from build123d import *

# Parameters (mm, degrees)
F1_DEPTH = 10
F3_D     = 3.4
F4_R     = 3


with BuildPart() as f1:
    # F0 (on Top) → F1 (new body, symmetric)
    with BuildSketch(Plane.XY):
        with BuildLine():
            ThreePointArc((-2, -12.338963), (0, 12.5), (2, -12.338963))
            Line((2, -12.338963), (2, -25))
            Line((2, -25), (30, -25))
            Line((30, -25), (30, -15))
            Line((30, -15), (17.5, -15))
            Line((17.5, -15), (17.5, 0))
            ThreePointArc((17.5, 0), (0, 17.5), (-17.5, 0))
            Line((-17.5, 0), (-17.5, -15))
            Line((-17.5, -15), (-30, -15))
            Line((-30, -15), (-30, -25))
            Line((-30, -25), (-2, -25))
            Line((-2, -25), (-2, -12.338963))
        make_face()
    extrude(amount=F1_DEPTH, both=True)

    # F3 (through all)
    with Locations(Plane(origin=(0, -15, 0), x_dir=(-1, 0, 0), z_dir=(0, 1, 0))):
        with Locations((24, 0), (-24, 0)):
            Hole(F3_D / 2)

    # F4
    f4_edges = [f1.edges().sort_by_distance(p)[0] for p in [
        (17.5, -15, 0),
        (-17.5, -15, 0),
        (-30, -20, 10),
        (-30, -20, -10),
        (30, -20, 10),
        (30, -20, -10),
    ]]
    fillet(f4_edges, radius=F4_R)


solid = f1.part
Design review of the part built by this model. Coordinates are the model's own, in mm. A direction names the side the tool comes from. Give positions to 0.01 mm unless a question says otherwise; leave off trailing zeros. Loops run counter-clockwise (first coordinate to the right, second up) from the corner with the lowest first, then second, coordinate; pieces in that order, holes last. Notation, with made-up numbers: M 40.25,68 L 83.25,68 A27 cw 83.25,100 Z; hole C 33.5,18.25 d8. An arc over 180 degrees is marked long. One line per question, with ' | ' between items. Start each with the question number.
1. The part is to be moulded in two halves that separate along X. For faces 1 (the face through (-0.52, 12.49, 0.14)), 2 (the face through (29.1, -19.93, 9.14)), 3 (the face through (-29.1, -20.07, -9.14)), say which applies: released by +X, released by -X, zero draft, split by the parting line, or undercut.
2. To check wall thickness, follow L1, parallel to Z at x = 24, y = -16.5; L2, parallel to X at y = -15.5, z = 5.75; L3, parallel to X at y = -7.5, z = -0.25. State the ranges of each line that lie inside material, in increasing order.
3. Add section B-B (x = 24). Write out the cut boundary in (y, z), plus the area to 3 significant figures.
4. Insertion check: P1, Ø5, axis at x = -23, z = -2.5, coming from the +Y side; P2, Ø12, axis at y = -13, z = -3, coming from the -X side; P3, Ø7.5, axis at x = 23, z = -0.5, coming from the +Y side; P4, Ø4, axis at y = -2.5, z = -3, coming from the +X side. Each pin has a flat end and moves straight along its axis. Give the tip position at first contact, or say it passes through.
5. For faces 4 (the face through (2, -19, 0)), 5 (the face through (-17.5, -6, 0)), 6 (the face through (25.57, -20.07, -0.65)), 7 (the face through (17.5, -6, 0)), list the 3-axis set-ups (+Z, -Z, +X, -X, +Y, -Y) from which the entire face can be reached by the end or side of a thin tool; tool diameter is ignored.
6. Add section A-A (y = -19). Write out the cut boundary in (x, z), plus the area to 3 significant figures.
7. Add section C-C (z = 0). Write out the cut boundary in (x, y).
8. Add section D-D (z = 5.25). Write out the cut boundary in (x, y), plus the area to 3 significant figures.
Worked out:
1) face 1: undercut | face 2: released by +X | face 3: released by -X
2) L1: z = -10 to -1.7, 1.7 to 10 | L2: x = -30 to -2, 2 to 30 | L3: x = -17.5 to -10, 10 to 17.5
3) outline: M -25,-10 L -15,-10 L -15,-1.7 L -25,-1.7 Z; M -25,1.7 L -15,1.7 L -15,10 L -25,10 Z | area: 166 mm²
4) P1: stops at y = -15 | P2: stops at x = -30 | P3: stops at y = -14.73 | P4: stops at x = 17.5
5) face 4: +Z, -Z, -Y | face 5: +Z, -Z, -X, +Y | face 6: +Y, -Y | face 7: +Z, -Z, +X, +Y
6) outline: M -30,-7 A3 ccw -27,-10 L -2,-10 L -2,10 L -27,10 A3 ccw -30,7 Z; M 2,-10 L 27,-10 A3 ccw 30,-7 L 30,7 A3 ccw 27,10 L 2,10 Z; hole C -24,0 d3.4; hole C 24,0 d3.4 | area: 1,090 mm²
7) outline: M -30,-25 L -25.7,-25 L -25.7,-15 L -30,-15 Z; M -22.3,-25 L -2,-25 L -2,-12.34 A12.5 cw long 2,-12.34 L 2,-25 L 22.3,-25 L 22.3,-15 L 20.5,-15 A3 cw 17.5,-12 L 17.5,0 A17.5 ccw -17.5,0 L -17.5,-12 A3 cw -20.5,-15 L -22.3,-15 Z; M 25.7,-25 L 30,-25 L 30,-15 L 25.7,-15 Z
8) outline: M -30,-25 L -2,-25 L -2,-12.34 A12.5 cw long 2,-12.34 L 2,-25 L 30,-25 L 30,-15 L 20.5,-15 A3 cw 17.5,-12 L 17.5,0 A17.5 ccw -17.5,0 L -17.5,-12 A3 cw -20.5,-15 L -30,-15 Z | area: 1,070 mm²
